Read the model definition and answer for the solid it produces. Units are mm, in the model's axes. Face numbers are marked on the shaded views. A direction names the side the tool comes from. Coordinates: 2 decimals unless noted, no trailing zeros. Order: outer loops, then holes, each group sorted by start corner. A loop starts at its lowest first (then second) coordinate and runs counter-clockwise, first axis right, second up. Notation, with made-up numbers: (48, 63.5) -> (85, 63.5) arc R30 ccw to (85, 85.5) -> close; hole circle Ø2 at (72.5, 60). An arc over 180 degrees is marked (long way). Return JSON: item names as keys, results as strings. Group by question number.
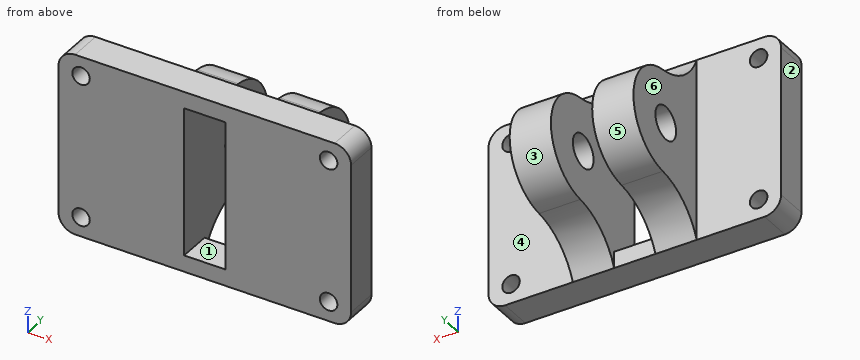
```python
from build123d import *

# Parameters (mm, degrees)
SKETCH1_W           = 45.0088
SKETCH1_H           = 27.9908
BOSS_EXTRUDE1_DEPTH = 5.0038
SKETCH2_R           = 1.3462
CUT_EXTRUDE1_DEPTH  = 5.0038
FILLET1_R           = 2.54
BOSS_EXTRUDE2_START = 3.175
SKETCH3_R           = 7.9375
SKETCH3_R_2         = 2.54
BOSS_EXTRUDE2_DEPTH = 6.35
BOSS_EXTRUDE3_START = -9.525
SKETCH4_R           = 7.9375
SKETCH4_R_2         = 2.54
BOSS_EXTRUDE3_DEPTH = 6.35
FILLET2_R           = 10.000000066
SKETCH5_W           = 6.35
SKETCH5_H           = 22.9108
CUT_EXTRUDE2_DEPTH  = 56.238689053


with BuildPart() as part:
    # Sketch1 → Boss-Extrude1 (new body)
    with BuildSketch(Plane(origin=(0, 0, 0), x_dir=(1, 0, 0), z_dir=(0, 1, 0))):
        with Locations((22.5044, 13.9954)):
            Rectangle(SKETCH1_W, SKETCH1_H)
    extrude(amount=BOSS_EXTRUDE1_DEPTH)

    # Sketch2 → Cut-Extrude1 (cut)
    with BuildSketch(Plane(origin=(0, 5.0038, 0), x_dir=(1, 0, 0), z_dir=(0, 1, 0))):
        with Locations(Location((41.5544, 24.9936, 0), (0, 0, 270))):
            Circle(SKETCH2_R)
        with Locations(Location((41.5544, 2.9972, 0), (0, 0, 90))):
            Circle(SKETCH2_R)
        with Locations(Location((3.4544, 24.9936, 0), (0, 0, 90))):
            Circle(SKETCH2_R)
        with Locations(Location((3.4544, 2.9972, 0), (0, 0, 270))):
            Circle(SKETCH2_R)
    extrude(amount=-CUT_EXTRUDE1_DEPTH, mode=Mode.SUBTRACT)

    # Fillet1
    fillet1_edges = [part.edges().sort_by_distance(p)[0] for p in [
        (0, 2.5019, -27.9908),
        (45.0088, 2.5019, -27.9908),
        (45.0088, 2.5019, 0),
        (0, 2.5019, 0),
    ]]
    fillet(fillet1_edges, radius=FILLET1_R)

    # Sketch3 → Boss-Extrude2 (add)
    with BuildSketch(Plane(origin=(22.5044, 0, 0), x_dir=(0, 0, -1), z_dir=(1, 0, 0)).offset(BOSS_EXTRUDE2_START)):
        with Locations((13.9954, 12.6238)):
            Circle(SKETCH3_R)
        with Locations((13.9954, 12.6238)):
            Circle(SKETCH3_R_2, mode=Mode.SUBTRACT)
    extrude(amount=BOSS_EXTRUDE2_DEPTH)

    # Sketch4 → Boss-Extrude3 (add)
    with BuildSketch(Plane(origin=(22.5044, 0, 0), x_dir=(0, 0, -1), z_dir=(1, 0, 0)).offset(BOSS_EXTRUDE3_START)):
        with Locations((13.9954, 12.6238)):
            Circle(SKETCH4_R)
        with Locations((13.9954, 12.6238)):
            Circle(SKETCH4_R_2, mode=Mode.SUBTRACT)
    extrude(amount=BOSS_EXTRUDE3_DEPTH)

    # Fillet2
    # the kernel refuses this fillet: 10.000000066 mm, written as the material it adds along each edge
    with BuildSketch(Plane(origin=(32.0294, 5.0038, -16.2179), x_dir=(0, 0, -1), z_dir=(-1, 0, 0)), Plane(origin=(19.3294, 5.0038, -16.2179), x_dir=(0, 0, -1), z_dir=(-1, 0, 0))) as fillet2_piece_1:
        with BuildLine():
            CenterArc((15.643447864, -9.220567258), FILLET2_R, 112.771363132, 62.10931252)
            Line((5.683337527, -8.328264951), (5.484135321, -8.310418905))
            ThreePointArc((5.484135321, -8.310418905), (4.168656518, -3.258575394), (-0.056, -0.192000001))
            Line((-0.056, -0.192000001), (0, 0.200000001))
            ThreePointArc((0, 0.200000001), (5.88645, 0.200000001), (11.695489043, 0.184411345))
            Line((11.695489043, 0.184411345), (11.7729, 0))
        make_face()
    extrude(amount=6.35)
    with BuildSketch(Plane(origin=(32.0294, 5.0038, -16.2179), x_dir=(0, 0, -1), z_dir=(-1, 0, 0))) as fillet2_piece_2_section:
        with BuildLine():
            CenterArc((15.643447864, -9.220567258), FILLET2_R, 112.771363132, 62.10931252)
            Line((5.683337527, -8.328264951), (5.484135321, -8.310418905))
            ThreePointArc((5.484135321, -8.310418905), (4.168656518, -3.258575394), (-0.056, -0.192000001))
            Line((-0.056, -0.192000001), (0, 0.200000001))
            ThreePointArc((0, 0.200000001), (5.88645, 0.200000001), (11.695489043, 0.184411345))
            Line((11.695489043, 0.184411345), (11.7729, 0))
        make_face()
    fillet2_piece_2 = extrude(amount=35.78225, mode=Mode.PRIVATE)
    fillet2_piece_2 = split(fillet2_piece_2, bisect_by=Plane(origin=(12.9794, 6.888894544, -22.053995201), z_dir=(1, 0, 0)), keep=Keep.TOP, mode=Mode.PRIVATE)
    fillet2_piece_2 = split(fillet2_piece_2, bisect_by=Plane(origin=(19.3294, 6.888894544, -22.053995201), z_dir=(-1, 0, 0)), keep=Keep.TOP, mode=Mode.PRIVATE)
    add(fillet2_piece_2)
    with BuildSketch(Plane(origin=(32.0294, 5.0038, -11.7729), x_dir=(0, 0, 1), z_dir=(-1, 0, 0)), Plane(origin=(19.3294, 5.0038, -11.7729), x_dir=(0, 0, 1), z_dir=(-1, 0, 0))) as fillet2_piece_3:
        with BuildLine():
            CenterArc((15.643447864, 9.220567258), FILLET2_R, 185.119324348, 62.10931252)
            Line((5.683337527, 8.328264951), (5.484135321, 8.310418905))
            ThreePointArc((5.484135321, 8.310418905), (4.168656518, 3.258575394), (-0.056, 0.192000001))
            Line((-0.056, 0.192000001), (0, -0.200000001))
            ThreePointArc((0, -0.200000001), (5.88645, -0.200000001), (11.695489043, -0.184411345))
            Line((11.695489043, -0.184411345), (11.7729, 0))
        make_face()
    extrude(amount=6.35)
    with BuildSketch(Plane(origin=(32.0294, 5.0038, -11.7729), x_dir=(0, 0, 1), z_dir=(-1, 0, 0))) as fillet2_piece_4_section:
        with BuildLine():
            CenterArc((15.643447864, 9.220567258), FILLET2_R, 185.119324348, 62.10931252)
            Line((5.683337527, 8.328264951), (5.484135321, 8.310418905))
            ThreePointArc((5.484135321, 8.310418905), (4.168656518, 3.258575394), (-0.056, 0.192000001))
            Line((-0.056, 0.192000001), (0, -0.200000001))
            ThreePointArc((0, -0.200000001), (5.88645, -0.200000001), (11.695489043, -0.184411345))
            Line((11.695489043, -0.184411345), (11.7729, 0))
        make_face()
    fillet2_piece_4 = extrude(amount=35.78225, mode=Mode.PRIVATE)
    fillet2_piece_4 = split(fillet2_piece_4, bisect_by=Plane(origin=(12.9794, 6.888894544, -5.936804799), z_dir=(1, 0, 0)), keep=Keep.TOP, mode=Mode.PRIVATE)
    fillet2_piece_4 = split(fillet2_piece_4, bisect_by=Plane(origin=(19.3294, 6.888894544, -5.936804799), z_dir=(-1, 0, 0)), keep=Keep.TOP, mode=Mode.PRIVATE)
    add(fillet2_piece_4)
    with BuildSketch(Plane(origin=(48.76165, 5.0038, -11.7729), x_dir=(0, 0, 1), z_dir=(-1, 0, 0))) as fillet2_piece_5_section:
        with BuildLine():
            CenterArc((15.643447864, 9.220567258), FILLET2_R, 185.119324348, 62.10931252)
            Line((5.683337527, 8.328264951), (5.484135321, 8.310418905))
            ThreePointArc((5.484135321, 8.310418905), (4.168656518, 3.258575394), (-0.056, 0.192000001))
            Line((-0.056, 0.192000001), (0, -0.200000001))
            ThreePointArc((0, -0.200000001), (5.88645, -0.200000001), (11.695489043, -0.184411345))
            Line((11.695489043, -0.184411345), (11.7729, 0))
        make_face()
    fillet2_piece_5 = extrude(amount=35.78225, mode=Mode.PRIVATE)
    fillet2_piece_5 = split(fillet2_piece_5, bisect_by=Plane(origin=(25.6794, 6.888894544, -5.936804799), z_dir=(1, 0, 0)), keep=Keep.TOP, mode=Mode.PRIVATE)
    fillet2_piece_5 = split(fillet2_piece_5, bisect_by=Plane(origin=(32.0294, 6.888894544, -5.936804799), z_dir=(-1, 0, 0)), keep=Keep.TOP, mode=Mode.PRIVATE)
    add(fillet2_piece_5)
    with BuildSketch(Plane(origin=(48.76165, 5.0038, -16.2179), x_dir=(0, 0, -1), z_dir=(-1, 0, 0))) as fillet2_piece_6_section:
        with BuildLine():
            CenterArc((15.643447864, -9.220567258), FILLET2_R, 112.771363132, 62.10931252)
            Line((5.683337527, -8.328264951), (5.484135321, -8.310418905))
            ThreePointArc((5.484135321, -8.310418905), (4.168656518, -3.258575394), (-0.056, -0.192000001))
            Line((-0.056, -0.192000001), (0, 0.200000001))
            ThreePointArc((0, 0.200000001), (5.88645, 0.200000001), (11.695489043, 0.184411345))
            Line((11.695489043, 0.184411345), (11.7729, 0))
        make_face()
    fillet2_piece_6 = extrude(amount=35.78225, mode=Mode.PRIVATE)
    fillet2_piece_6 = split(fillet2_piece_6, bisect_by=Plane(origin=(25.6794, 6.888894544, -22.053995201), z_dir=(1, 0, 0)), keep=Keep.TOP, mode=Mode.PRIVATE)
    fillet2_piece_6 = split(fillet2_piece_6, bisect_by=Plane(origin=(32.0294, 6.888894544, -22.053995201), z_dir=(-1, 0, 0)), keep=Keep.TOP, mode=Mode.PRIVATE)
    add(fillet2_piece_6)

    # Sketch5 → Cut-Extrude2 (cut, through all)
    with BuildSketch(Plane(origin=(0, 5.0038, 0), x_dir=(1, 0, 0), z_dir=(0, 1, 0))):
        with Locations((22.5044, 13.9954)):
            Rectangle(SKETCH5_W, SKETCH5_H)
    extrude(amount=-CUT_EXTRUDE2_DEPTH, mode=Mode.SUBTRACT)


solid = part.part
```
1. Straight lines are drawn through the part: L1, parallel to X at y = 8.5, z = -18; L2, parallel to Z at x = 24, y = 2.5; L3, parallel to X at y = 3.75, z = -16.25. For each, find the intervals that lie inside material, in ascending order.
2. Given pin 1 (1.3 mm diameter, centred on x = 22.5, z = -1, fed in from +Y); pin 2 (8 mm diameter, centred on y = 11, z = -17, fed in from -X); pin 3 (8 mm diameter, centred on y = 12.62, z = -14, fed in from +X), each flat-ended and moving along its own axis, determine where each tip first touches the part or whether it passes through.
3. Find section D-D on y = 8.5. Determine the outline of the cut face in (x, z).
4. Find section B-B on x = 21.5. Determine the outline of the cut face in (y, z).
5. Which of the six approach directions +Z, -Z, +X, -X, +Y, -Y give full straight-line access (tool end or side, diameter ignored) to the marked faces 4, 5 and 6?
6. For a pull along Z with two mould halves and no side action, classify the marked faces 1, 2 and 3 as released by +Z, released by -Z, zero draft, split by the parting line, or undercut.
7. Find section A-A on z = -3.5. Determine the outline of the cut face in (x, y), and give its area (3 significant figures).
8. Find section C-C on y = 12. Determine the outline of the cut face in (x, z), and give its area (3 significant figures).
Result:
{
 "1": {"L1": "12.98 to 19.33, 25.68 to 32.03", "L2": "-27.99 to -25.45, -2.54 to 0", "L3": "0 to 19.33, 25.68 to 45.01"},
 "2": {"pin 1": "y = 5", "pin 2": "x = 12.98", "pin 3": "x = 32.03"},
 "3": {"outline": "(12.98, -23.66) -> (19.33, -23.66) -> (19.33, -4.33) -> (12.98, -4.33) -> close; (25.68, -23.66) -> (32.03, -23.66) -> (32.03, -4.33) -> (25.68, -4.33) -> close"},
 "4": {"outline": "(0, -27.99) -> (5, -27.99) -> (5, -25.45) -> (0, -25.45) -> close; (0, -2.54) -> (5, -2.54) -> (5, 0) -> (0, 0) -> close"},
 "5": {"face 4": "+Z, -Z, +X, +Y", "face 5": "+X, -X, +Y", "face 6": "+Z, -Z, -X, +Y"},
 "6": {"face 1": "undercut", "face 2": "zero draft", "face 3": "split by the parting line"},
 "7": {"outline": "(0, 0) -> (2.21, 0) -> (2.21, 5) -> (0, 5) -> close; (4.7, 0) -> (19.33, 0) -> (19.33, 7.47) -> (12.98, 7.47) -> (12.98, 5) -> (4.7, 5) -> close; (25.68, 0) -> (40.31, 0) -> (40.31, 5) -> (32.03, 5) -> (32.03, 7.47) -> (25.68, 7.47) -> close; (42.8, 0) -> (45.01, 0) -> (45.01, 5) -> (42.8, 5) -> close", "area": "200 mm^2"},
 "8": {"outline": "(12.98, -22.11) -> (19.33, -22.11) -> (19.33, -16.46) -> (12.98, -16.46) -> close; (12.98, -11.53) -> (19.33, -11.53) -> (19.33, -5.88) -> (12.98, -5.88) -> close; (25.68, -22.11) -> (32.03, -22.11) -> (32.03, -16.46) -> (25.68, -16.46) -> close; (25.68, -11.53) -> (32.03, -11.53) -> (32.03, -5.88) -> (25.68, -5.88) -> close", "area": "144 mm^2"}
}
